```python
from build123d import *

# Parameters (mm, degrees)
F1_DEPTH = 15.8
F2_W     = 20
F2_H     = 3
F3_DEPTH = 2.7
F4_W     = 15
F4_H     = 15.8
F5_DEPTH = 5.5
F6_R     = 2
F7_DEPTH = 15.801


with BuildPart() as f1:
    # F0 (on Front) → F1 (new body)
    with BuildSketch(Plane.XZ):
        Polygon((-25.9, -20), (-25.9, 0), (25.9, 0), (25.9, -20), (29.9, -20), (29.9, 4), (-29.9, 4), (-29.9, -20), align=None)
    extrude(amount=F1_DEPTH)

    # F2 (on face) → F3 (join)
    with BuildSketch(Plane.XZ.offset(15.8)):
        with Locations((1.4, -1.5)):
            Rectangle(F2_W, F2_H)
    extrude(amount=-F3_DEPTH)

    # F4 (on face) → F5 (join)
    with BuildSketch(Plane.XY.offset(4)):
        with Locations((0, -7.9)):
            Rectangle(F4_W, F4_H)
    extrude(amount=F5_DEPTH)

    # F6 (on face) → F7 (cut, through all)
    with BuildSketch(Plane.XZ.offset(15.8)):
        with Locations((-24.52996, -1.37004)):
            Circle(F6_R)
        with Locations((24.52996, -1.37004)):
            Circle(F6_R)
    extrude(amount=-F7_DEPTH, mode=Mode.SUBTRACT)


solid = f1.part
```
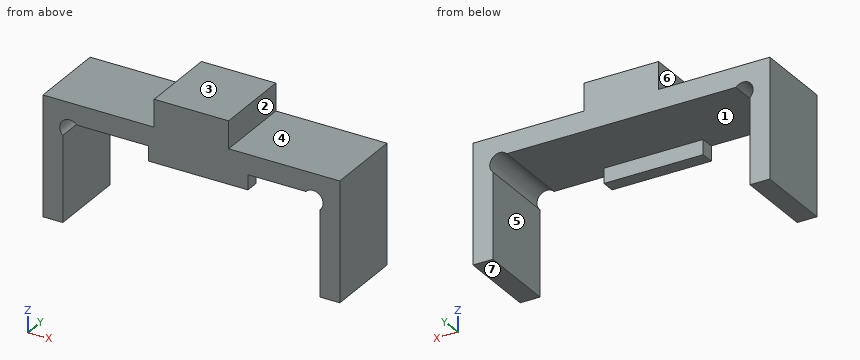
Here's how the part is built. I have some questions about the finished solid (model axes, mm). Face numbers are marked on the shaded views. A direction names the side the tool comes from. Give positions to 0.01 mm unless a question says otherwise; leave off trailing zeros. Loops run counter-clockwise (first coordinate to the right, second up) from the corner with the lowest first, then second, coordinate; pieces in that order, holes last. Notation, with made-up numbers: M 27,-4.75 L 63,-4.75 A15 cw 63,10.25 Z; hole C -8,-21 d4. An arc over 180 degrees is marked long. Return JSON: item names as keys, results as strings.
Item 1: Please list where these lines run through material, in increasing order: line 1 (X direction, y = -12.5, z = -4.25); line 2 (Z direction, x = -13.5, y = -6); line 3 (X direction, y = -5.5, z = 7.5).
A:
{"line 1": "x = -29.9 to -25.9, 25.9 to 29.9", "line 2": "z = 0 to 4", "line 3": "x = -7.5 to 7.5"}
Item 2: Imagine slicing it at C-C on x = -2. List the corners of the cut face in (y, z) for me.
A:
{"outline": "M -15.8,-3 L -13.1,-3 L -13.1,0 L 0,0 L 0,9.5 L -15.8,9.5 Z"}
Item 3: Imagine slicing it at A-A on z = -5.25. List the corners of the cut face in (x, y) for me.
A:
{"outline": "M -29.9,-15.8 L -25.9,-15.8 L -25.9,0 L -29.9,0 Z; M 25.9,-15.8 L 29.9,-15.8 L 29.9,0 L 25.9,0 Z"}
Item 4: On a 3-axis mill with a long thin cutter (end or side, diameter ignored), from which of +Z, -Z, +X, -X, +Y, -Y can I reach the whole of each face in a straight line? I mean the marked faces 4, 5, 6 and 7. Say none if no direction works.
A:
{"face 4": "+Z, +X, +Y, -Y", "face 5": "-Z, +Y, -Y", "face 6": "+Z, -X, +Y, -Y", "face 7": "-Z, +X, -X, +Y, -Y"}
Item 5: Imagine slicing it at D-D on z = 5.5. List the corners of the cut face in (x, y) for me, then the cut area to 3 significant figures.
A:
{"outline": "M -7.5,-15.8 L 7.5,-15.8 L 7.5,0 L -7.5,0 Z", "area": "237 mm^2"}
Item 6: I'm going to push flat-ended pins straight in: pin 1 Ø5 at (x, y) = (-20.5, -3.5) entering from -Z; pin 2 Ø3 at (y, z) = (-12, 7) entering from +X; pin 3 Ø4.5 at (y, z) = (-6, 6.5) entering from -X. Where does each tip first touch, or does it pass through?
A:
{"pin 1": "stops at z = 0", "pin 2": "stops at x = 7.5", "pin 3": "stops at x = -7.5"}
Item 7: Thinking about a two-plate mould opening in X: for the marked faces 1, 2 and 3, which applies, released by +X, released by -X, zero draft, split by the parting line, or undercut?
A:
{"face 1": "undercut", "face 2": "released by +X", "face 3": "zero draft"}
Item 8: Imagine slicing it at B-B on y = -14. List the corners of the cut face in (x, z) for me, then the cut area to 3 significant figures.
A:
{"outline": "M -29.9,-20 L -25.9,-20 L -25.9,-2.83 A2 cw long -23.07,0 L -8.6,0 L -8.6,-3 L 11.4,-3 L 11.4,0 L 23.07,0 A2 cw long 25.9,-2.83 L 25.9,-20 L 29.9,-20 L 29.9,4 L 7.5,4 L 7.5,9.5 L -7.5,9.5 L -7.5,4 L -29.9,4 Z", "area": "537 mm^2"}
